Part model, mm, in its own coordinate system. A direction names the side the tool comes from. Give positions to 0.01 mm unless a question says otherwise; leave off trailing zeros. Loops run counter-clockwise (first coordinate to the right, second up) from the corner with the lowest first, then second, coordinate; pieces in that order, holes last. Notation, with made-up numbers: (30, -2.75) -> (72, -2.75) arc R25 cw to (72, 17.25) -> close; hole circle Ø3 at (30, 58.5). An arc over 180 degrees is marked (long way). One line per question, with ' | ' between items.
```python
from build123d import *

# Parameters (mm, degrees)
CROQUIS1_R              = 11
CROQUIS1_W              = 12
CROQUIS1_H              = 10
SALIENTE_EXTRUIR1_DEPTH = 26
CROQUIS3_R              = 11
CROQUIS3_R_2            = 8
SALIENTE_EXTRUIR2_DEPTH = 30
CROQUIS5_R              = 11
CROQUIS5_R_2            = 5
SALIENTE_EXTRUIR3_DEPTH = 15


with BuildPart() as part:
    # Croquis1 → Saliente-Extruir1 (new body)
    with BuildSketch(Plane.XY):
        Circle(CROQUIS1_R)
        Rectangle(CROQUIS1_W, CROQUIS1_H, mode=Mode.SUBTRACT)
    extrude(amount=SALIENTE_EXTRUIR1_DEPTH)

    # Croquis3 → Saliente-Extruir2 (add)
    with BuildSketch(Plane.XY.offset(26)):
        Circle(CROQUIS3_R)
        Circle(CROQUIS3_R_2, mode=Mode.SUBTRACT)
    extrude(amount=SALIENTE_EXTRUIR2_DEPTH)

    # Croquis5 → Saliente-Extruir3 (add)
    with BuildSketch(Plane.XY.offset(56)):
        Circle(CROQUIS5_R)
        Circle(CROQUIS5_R_2, mode=Mode.SUBTRACT)
    extrude(amount=-SALIENTE_EXTRUIR3_DEPTH)


solid = part.part
```
1) Saw through at B-B (y = 0). Give the cut face in (x, z), and give its area (3 significant figures).
Found:
outline: (-11, 0) -> (-6, 0) -> (-6, 26) -> (-8, 26) -> (-8, 41) -> (-5, 41) -> (-5, 56) -> (-11, 56) -> close; (5, 41) -> (8, 41) -> (8, 26) -> (6, 26) -> (6, 0) -> (11, 0) -> (11, 56) -> (5, 56) -> close | area: 530 mm2
2) Drill centre lines: line 1 (Z direction, x = 4.25, y = -6.5); line 2 (Y direction, x = 0, z = 50.25); line 3 (Y direction, x = -0.25, z = 36). Where is each one in solid material? Low to high.
Found:
line 1: 0 to 26, 41 to 56 | line 2: -11 to -5, 5 to 11 | line 3: -11 to -8, 8 to 11
3) Saw through at A-A (x = 0). Give the cut face in (y, z), and give its area (3 significant figures).
Found:
outline: (-11, 0) -> (-5, 0) -> (-5, 26) -> (-8, 26) -> (-8, 41) -> (-5, 41) -> (-5, 56) -> (-11, 56) -> close; (5, 0) -> (11, 0) -> (11, 56) -> (5, 56) -> (5, 41) -> (8, 41) -> (8, 26) -> (5, 26) -> close | area: 582 mm2
4) Pull direction X, two halves, no side cores. Call faces 1 (the flat face through (6, 0, 13)), 2 (the flat face through (-6, 0, 13)), 3 (the flat face through (7, 0, 0)), 4 (the cylindrical face through (-2.38, -10.74, 27.61)): pulls with the +X half, pulls with the -X half, needs draft (parallel to the pull), parting line crosses it, or undercut.
Found:
face 1: undercut | face 2: undercut | face 3: needs draft | face 4: parting line crosses it
5) Tool access for faces 5 (the cylindrical face through (-1.08, -4.88, 48.6)), 6 (the flat face through (-0.1, -5.2, 26)), 7 (the flat face through (0, 5, 13)): list every direction of +Z, -Z, +X, -X, +Y, -Y with a clear straight run to the whole face (end or side of a thin tool).
Found:
face 5: +Z, -Z | face 6: none | face 7: -Z
6) Saw through at D-D (y = 5.75). Give the cut face in (x, z), and give its area (3 significant figures).
Found:
outline: (-9.38, 0) -> (9.38, 0) -> (9.38, 56) -> (-9.38, 56) -> close; hole (-5.56, 26) -> (5.56, 26) -> (5.56, 41) -> (-5.56, 41) -> close | area: 883 mm2
7) Pin check, flat tips, straight feed: P1, Ø3.5, axis at x = 2.5, z = 14.5, coming from the +Y side; P2, Ø8, axis at x = 1.5, z = 8.5, coming from the -Y side; P3, Ø1.5, axis at x = 5, z = 19, coming from the -Y side; P4, Ø5, axis at x = -6.5, z = 11, coming from the -Y side. Stop position of each tip, or through.
Found:
P1: y = 10.97 | P2: y = -11 | P3: y = -10.15 | P4: y = -10.25
8) Saw through at C-C (z = 52.5). Give the cut face in (x, y), and give its area (3 significant figures).
Found:
outline: circle Ø22 at (0, 0); hole circle Ø10 at (0, 0) | area: 302 mm2
